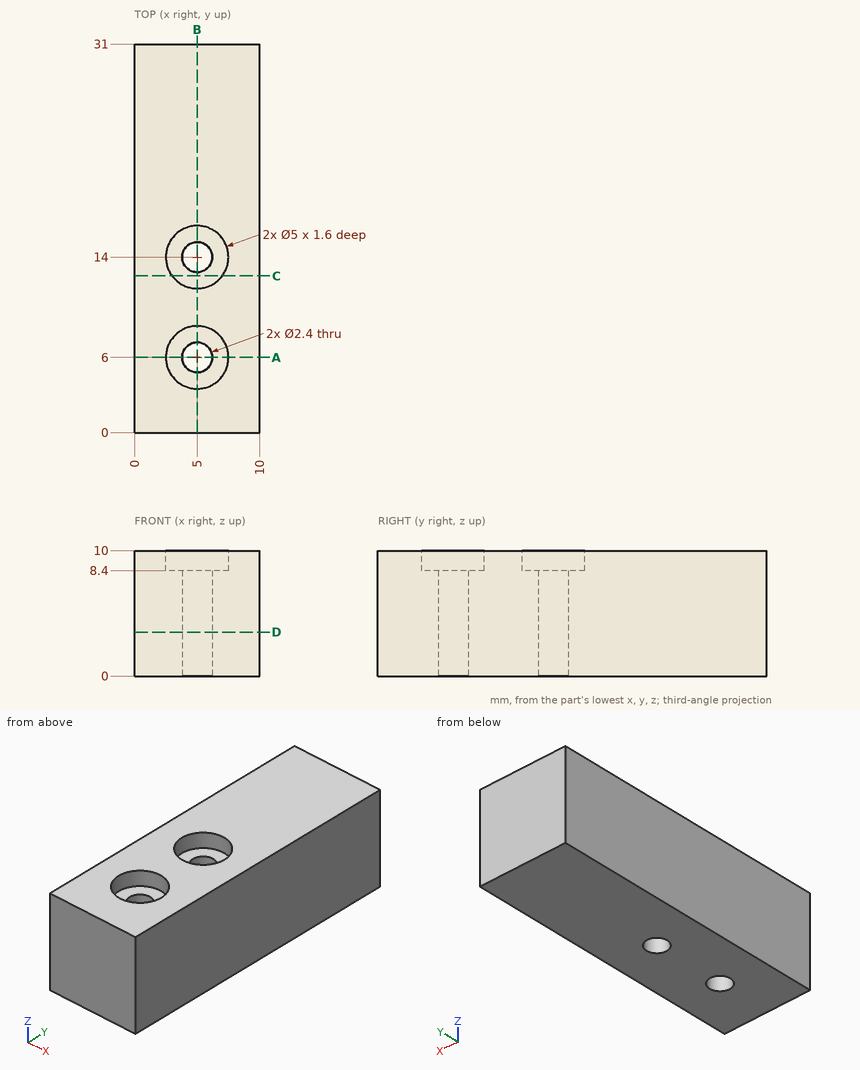
Design review of the part shown in the three views and the two pictorial views. Dimensions are in mm from the part's minimum x, y and z. Give positions to 0.01 mm unless a question says otherwise; leave off trailing zeros. Write each loop counter-clockwise with the first axis right and the second up, starting at its lowest first coordinate (ties: lowest second). Pieces come first, ordered by that corner, then holes. Notation, with made-up numbers: M -30.75,21.25 L 5.25,21.25 A22 cw 5.25,44.25 Z; hole C 84,73.5 d1. An arc over 180 degrees is marked long. One line per item, written item: value.
1) For P1, Ø4, axis at x = 5, y = 15, coming from the +Z side; P2, Ø2, axis at x = 5, y = 6, coming from the +Z side, all flat-tipped, find the tip position at first contact; note any pin that passes through.
Results are:
P1: stops at z = 10
P2: passes through
2) Take a section at C-C, the plane y = 12.5. Write out the cut boundary in (x, z).
Results are:
outline: M 0,0 L 10,0 L 10,10 L 7,10 L 7,8.4 L 3,8.4 L 3,10 L 0,10 Z
3) Take a section at B-B, the plane x = 5. Write out the cut boundary in (y, z), then the cut area to 3 significant figures.
Results are:
outline: M 0,0 L 4.8,0 L 4.8,8.4 L 3.5,8.4 L 3.5,10 L 0,10 Z; M 7.2,0 L 12.8,0 L 12.8,8.4 L 11.5,8.4 L 11.5,10 L 8.5,10 L 8.5,8.4 L 7.2,8.4 Z; M 15.2,0 L 31,0 L 31,10 L 16.5,10 L 16.5,8.4 L 15.2,8.4 Z
area: 254 mm²
4) Take a section at D-D, the plane z = 3.5. Write out the cut boundary in (x, y), then the cut area to 3 significant figures.
Results are:
outline: M 0,0 L 10,0 L 10,31 L 0,31 Z; hole C 5,6 d2.4; hole C 5,14 d2.4
area: 301 mm²
5) For line 1 (Y direction, x = 5, z = 4.25); line 2 (Y direction, x = 5, z = 9.65); line 3 (X direction, y = 14, z = 2), list the stretches that pass through material, from the lowest coordinate up. Write a range as from..to.
Results are:
line 1: y = 0..4.8, 7.2..12.8, 15.2..31
line 2: y = 0..3.5, 8.5..11.5, 16.5..31
line 3: x = 0..3.8, 6.2..10
6) Take a section at A-A, the plane y = 6. Write out the cut boundary in (x, z).
Results are:
outline: M 0,0 L 3.8,0 L 3.8,8.4 L 2.5,8.4 L 2.5,10 L 0,10 Z; M 6.2,0 L 10,0 L 10,10 L 7.5,10 L 7.5,8.4 L 6.2,8.4 Z
